Geometry check sheet. Reference: drawing and pictorial views, mm from the part's lowest x, y, z. Give positions to 0.01 mm unless a question says otherwise; leave off trailing zeros. Loops run counter-clockwise (first coordinate to the right, second up) from the corner with the lowest first, then second, coordinate; pieces in that order, holes last. Notation, with made-up numbers: (38.5, 24.25) -> (88.5, 24.25) arc R27 cw to (88.5, 46.25) -> close; hole circle Ø6 at (-2.5, -22.75). An arc over 180 degrees is marked (long way). Write item = value, one per line. Start each with the question number.
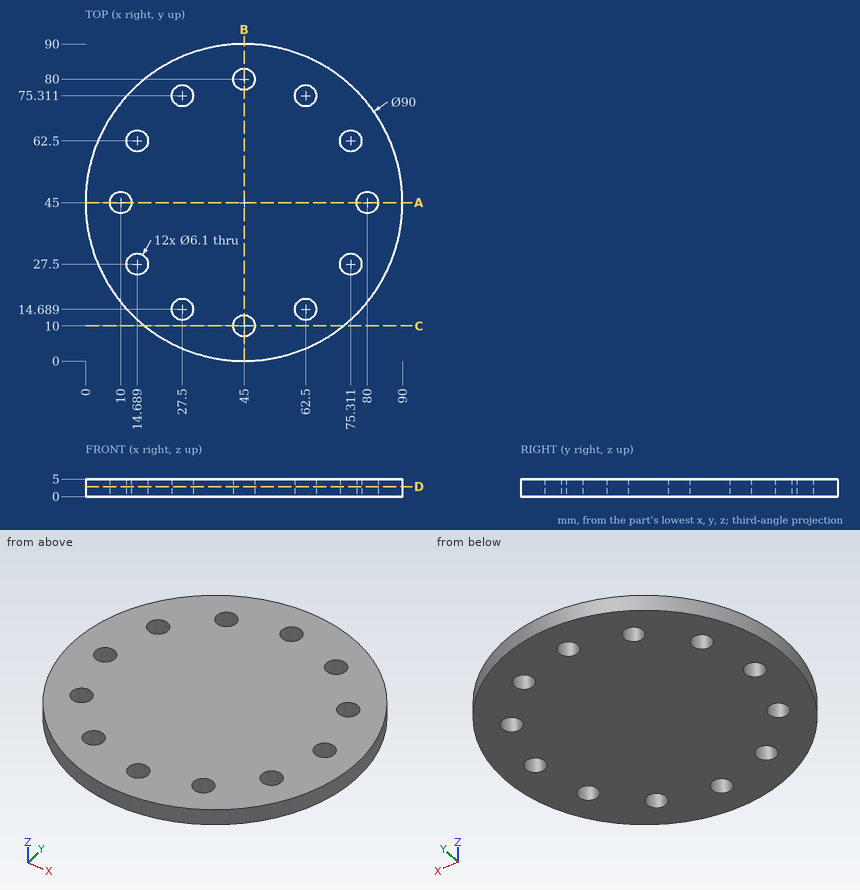
1) Section check D-D (z = 2.8). Give the number of separate pieces and of enclosed holes in the cut face, plus the area to 3 significant figures.
2) Thickness scan on line 1 (X direction, y = 74, z = 0.75); line 2 (Y direction, x = 27.5, z = 2.85); line 3 (X direction, y = 15.5, z = 1.65). Record the ranges inside material, lowest first.
3) Section check C-C (y = 10). Enter the section's corners in (x, z).
4) Depth check by flat-ended pin: pin 1 Ø7 at (x, y) = (10, 45) entering from -Z; pin 2 Ø2 at (y, z) = (76, 1) entering from -X; pin 3 Ø2 at (y, z) = (49.5, 3.5) entering from -X. Enter the tip coordinate at first touch or a pass-through.
5) Section check A-A (y = 45). Enter the section's corners in (x, z), plus the area to 3 significant figures.
Check result:
q1.separate_pieces = 1
q1.enclosed_holes = 12
q1.area = 6,010 mm2
q2.line_1 = 10.59 to 24.75, 30.25 to 59.75, 65.25 to 79.41
q2.line_2 = 3.54 to 11.64, 17.74 to 72.26, 78.36 to 86.46
q2.line_3 = 11.02 to 24.56, 30.44 to 59.56, 65.44 to 78.98
q3.outline = (16.72, 0) -> (41.95, 0) -> (41.95, 5) -> (16.72, 5) -> close; (48.05, 0) -> (73.28, 0) -> (73.28, 5) -> (48.05, 5) -> close
q4.pin_1 = 0
q4.pin_2 = 11.46
q4.pin_3 = 0.14
q5.outline = (0, 0) -> (6.95, 0) -> (6.95, 5) -> (0, 5) -> close; (13.05, 0) -> (76.95, 0) -> (76.95, 5) -> (13.05, 5) -> close; (83.05, 0) -> (90, 0) -> (90, 5) -> (83.05, 5) -> close
q5.area = 389 mm2
